Read the model definition and answer for the solid it produces. Units are mm, in the model's axes. A direction names the side the tool comes from. Round coordinates to 2 decimals unless told otherwise and drop trailing zeros. Order: outer loops, then holes, each group sorted by start corner. A loop starts at its lowest first (then second) coordinate and runs counter-clockwise, first axis right, second up. Notation, with made-up numbers: (-25, -21.75) -> (20, -21.75) arc R25 cw to (20, -6.75) -> close; hole circle Ø6 at (-22.75, 62). An arc over 180 degrees is marked (long way). One line per item, written item: value. Start each with the question number.
1. Section D-D (z = 30.5) is taken. Give the vertices of the cut face in (x, y), then the cut area to 3 significant figures.
2. The mould has two halves that part along X. Classify faces 4 (the face through (2.399, 15.385, 4.141)), 5 (the face through (1, 17, 1.6)), 6 (the face through (-3, 18.3, 34.4)): released by +X, released by -X, zero draft, split by the parting line, or undercut.
3. Consider line 1 (Y direction, x = 0, z = 3); line 2 (Y direction, x = 0, z = 0.5); line 3 (X direction, y = 20.25, z = 32). Determine where each line is inside the solid, lowest interval first.
4. For faces 1 (the face through (-3, 20.715, 20)), 2 (the face through (-3, 15.915, 20)), 3 (the face through (-2.2, 18, 21)), determine the directions among +Z, -Z, +X, -X, +Y, -Y from which every point of the face is accessible in a straight line to the end or side of a thin tool.
5. Flat-ended cylindrical pins translate along their axes: pin 1 Ø1.3 at (x, z) = (-3, 21.5) entering from +Y; pin 2 Ø4 at (y, z) = (18.5, 27.5) entering from +X; pin 3 Ø3 at (x, y) = (0, 18.23) entering from -Z. Find the tip coordinate at first contact, or state that the pin passes through.
6. Section A-A (x = 0) is taken. Give the vertices of the cut face in (y, z), then the cut area to 3 significant figures.
7. Section B-B (z = 4) is taken. Give the vertices of the cut face in (x, y).
8. Section C-C (x = -3.5) is taken. Give the vertices of the cut face in (y, z).
from build123d import *

# Parameters (mm, degrees)
F1_DEPTH  = 8.4
F2_R      = 2.5
F3_DEPTH  = 1.6
F4_R      = 1.25
F5_DEPTH  = 10
F6_W      = 2
F6_H      = 4.8
F7_DEPTH  = 26
F8_R      = 2
F9_DEPTH  = 0.2
F10_DEPTH = 0.2


# Not quite as in the source:
# - a feature names something its author has since deleted; it is built from what else it names


with BuildPart() as f1:
    # F0 (on Top) → F1 (new body)
    with BuildSketch(Plane.XY):
        with BuildLine():
            Line((1, 21.8148477226), (-4, 21.8148477226))
            Line((-4, 21.8148477226), (-4, 14.8148477226))
            Line((-4, 14.8148477226), (1, 14.8148477226))
            ThreePointArc((1, 14.8148477226), (2.4142135624, 15.4006341603), (3, 16.8148477226))
            Line((3, 16.8148477226), (3, 19.8148477226))
            ThreePointArc((3, 19.8148477226), (2.4142135624, 21.229061285), (1, 21.8148477226))
        make_face()
    extrude(amount=F1_DEPTH)

    # F2 (on face) → F3 (cut)
    with BuildSketch(Plane(origin=(0, 0, 0), x_dir=(1, 0, 0), z_dir=(0, 0, -1))):
        with Locations((0, -18.2346012443)):
            Circle(F2_R)
    extrude(amount=-F3_DEPTH, mode=Mode.SUBTRACT)

    # F4 (on face) → F5 (cut)
    with BuildSketch(Plane(origin=(0, 0, 1.6), x_dir=(1, 0, 0), z_dir=(0, 0, -1))):
        with Locations((0, -18.2346012443)):
            Circle(F4_R)
    extrude(amount=-F5_DEPTH, mode=Mode.SUBTRACT)

    # F6 (on face) → F7 (join)
    with BuildSketch(Plane.XY.offset(8.4)):
        with Locations((-3, 18.3148477226)):
            Rectangle(F6_W, F6_H)
    extrude(amount=F7_DEPTH)

    # F8
    f8_edges = [f1.edges().sort_by_distance(p)[0] for p in [
        (-3, 20.714848, 34.4),
        (-3, 15.914848, 34.4),
    ]]
    fillet(f8_edges, radius=F8_R)

    # F9 (cut): a face of the model
    f9_faces = [f1.faces().sort_by_distance(p)[0] for p in [
        (-2, 18.3148477226, 21.2249019293),
    ]]
    extrude(f9_faces, amount=-F9_DEPTH, mode=Mode.SUBTRACT)

    # F10 (cut): a face of the model
    f10_faces = [f1.faces().sort_by_distance(p)[0] for p in [
        (-4, 18.3148477226, 15.72101639),
    ]]
    extrude(f10_faces, amount=-F10_DEPTH, mode=Mode.SUBTRACT)


solid = f1.part
Answer:
1. outline: (-3.8, 15.91) -> (-2.2, 15.91) -> (-2.2, 20.71) -> (-3.8, 20.71) -> close
1. area: 7.68 mm^2
2. face 4: released by +X
2. face 5: undercut
2. face 6: zero draft
3. line 1: 14.81 to 16.98, 19.48 to 21.81
3. line 2: 14.81 to 15.73, 20.73 to 21.81
3. line 3: -3.8 to -2.2
4. face 1: +Z, +X, -X, +Y
4. face 2: +Z, +X, -X, -Y
4. face 3: +Z, +X, +Y, -Y
5. pin 1: y = 20.71
5. pin 2: x = -2.2
5. pin 3: z = 1.6
6. outline: (14.81, 0) -> (15.73, 0) -> (15.73, 1.6) -> (16.98, 1.6) -> (16.98, 8.4) -> (14.81, 8.4) -> close; (19.48, 1.6) -> (20.73, 1.6) -> (20.73, 0) -> (21.81, 0) -> (21.81, 8.4) -> (19.48, 8.4) -> close
6. area: 33.8 mm^2
7. outline: (-3.8, 14.81) -> (1, 14.81) arc R2 ccw to (3, 16.81) -> (3, 19.81) arc R2 ccw to (1, 21.81) -> (-3.8, 21.81) -> close; hole circle Ø2.5 at (0, 18.23)
8. outline: (14.81, 0) -> (21.81, 0) -> (21.81, 8.4) -> (20.71, 8.4) -> (20.71, 32.4) arc R2 ccw to (18.71, 34.4) -> (17.91, 34.4) arc R2 ccw to (15.91, 32.4) -> (15.91, 8.4) -> (14.81, 8.4) -> close
